from build123d import *

# Parameters (mm, degrees)
SKETCH2_R          = 10
CUT_EXTRUDE1_DEPTH = 216
CUT_EXTRUDE2_DEPTH = 108
CUT_EXTRUDE3_DEPTH = 108
SKETCH7_R          = 15
CUT_EXTRUDE4_DEPTH = 108


with BuildPart() as part:
    # Sketch1 → Revolve1 (revolve)
    with BuildSketch(Plane(origin=(0, 0, 0), x_dir=(1, 0, 0), z_dir=(0, 1, 0)), mode=Mode.PRIVATE) as revolve1_sk:
        Polygon((-1.846866082, -35.985748219), (-1.846866082, 124.014251781), (-46.846866082, 124.014251781), (-46.846866082, 34.014251781), (-31.846866082, 34.014251781), (-31.846866082, -5.985748219), (-21.846866082, -5.985748219), (-21.846866082, -35.985748219), align=None)
    revolve(revolve1_sk.sketch.rotate(Axis((-1.846866082, 0, 35.985748219), (0, 0, -1)), 180), axis=Axis((-1.846866082, 0, 35.985748219), (0, 0, -1)))

    # Sketch2 → Cut-Extrude1 (cut)
    with BuildSketch(Plane.XY.offset(35.985748219)):
        Circle(SKETCH2_R)
    extrude(amount=-CUT_EXTRUDE1_DEPTH, mode=Mode.SUBTRACT)

    # Sketch4 → Cut-Extrude2 (cut, symmetric)
    with BuildSketch(Plane(origin=(0, 0, 0), x_dir=(0, 0, -1), z_dir=(1, 0, 0))):
        with BuildLine():
            Line((124.014251781, 45), (64.014251781, 45))
            Line((64.014251781, 45), (64.014251781, 40))
            ThreePointArc((64.014251781, 40), (66.94318397, 32.928932188), (74.014251781, 30))
            Line((74.014251781, 30), (94.014251781, 30))
            ThreePointArc((94.014251781, 30), (115.227455222, 21.213203431), (124.014251781, -1.4e-08))
            Line((124.014251781, -1.4e-08), (124.014251781, 45))
        make_face()
        with BuildLine():
            Line((124.014251781, -45), (124.014251781, -1.4e-08))
            ThreePointArc((124.014251781, -1.4e-08), (115.227455212, -21.213203441), (94.014251781, -30))
            Line((94.014251781, -30), (74.014251781, -30))
            ThreePointArc((74.014251781, -30), (66.94318397, -32.928932188), (64.014251781, -40))
            Line((64.014251781, -40), (64.014251781, -45))
            Line((64.014251781, -45), (124.014251781, -45))
        make_face()
    extrude(amount=CUT_EXTRUDE2_DEPTH, both=True, mode=Mode.SUBTRACT)

    # Sketch5 → Cut-Extrude3 (cut, symmetric)
    with BuildSketch(Plane(origin=(0, -30, 0), x_dir=(-1, 0, 0), z_dir=(0, -1, 0))):
        with BuildLine():
            Line((-20, 129.367247505), (20, 129.367247505))
            Line((20, 129.367247505), (20, 79.367247505))
            ThreePointArc((20, 79.367247505), (17.071067812, 72.296179693), (10, 69.367247505))
            Line((10, 69.367247505), (-10, 69.367247505))
            ThreePointArc((-10, 69.367247505), (-17.071067812, 72.296179693), (-20, 79.367247505))
            Line((-20, 79.367247505), (-20, 129.367247505))
        make_face()
    extrude(amount=CUT_EXTRUDE3_DEPTH, both=True, mode=Mode.SUBTRACT)

    # Sketch7 → Cut-Extrude4 (cut, symmetric)
    with BuildSketch(Plane(origin=(0, 0, 0), x_dir=(0, 0, -1), z_dir=(1, 0, 0))):
        with Locations((94.014251781, 0)):
            Circle(SKETCH7_R)
    extrude(amount=CUT_EXTRUDE4_DEPTH, both=True, mode=Mode.SUBTRACT)


solid = part.part
Geometry: final body of the model. Coordinates: model frame, mm. A direction names the side the tool comes from. Coordinates: 2 decimals unless noted, no trailing zeros. Loops run counter-clockwise (first coordinate to the right, second up) from the corner with the lowest first, then second, coordinate; pieces in that order, holes last. Notation, with made-up numbers: (45.25, -37) - (89.25, -37) arc R24 cw to (89.25, -13) - close; hole circle Ø5 at (52.25, 31.25). An arc over 180 degrees is marked (long way). One line per question, with ' | ' between items. Start each with the question number.
(1) Reachability of faces 4 (the cylindrical face through (17.23, -6.01, 21.2)), 5 (the flat face through (25, 30, -84)), 6 (the flat face through (20, 0, -111)), 7 (the cylindrical face through (-33.23, 0.66, -79.03)) from +Z, -Z, +X, -X, +Y, -Y: full face, straight path, thin tool, end or side. Return the list, or none.
(2) Cut plane B-B on z = -96.5. Output: boundary loops of the cut face in (x, y), and give its area (3 significant figures).
(3) Cut plane D-D on z = -41. Output: boundary loops of the cut face in (x, y).
(4) Cut plane A-A on x = 1. Output: boundary loops of the cut face in (y, z).
(5) First-contact query: pin 1 (8 mm diameter, centred on y = -23.5, z = -64.5, fed in from +X); pin 2 (10.5 mm diameter, centred on x = 22, z = -83.5, fed in from -Y); pin 3 (1.5 mm diameter, centred on x = -8, y = -42.5, fed in from -Z). Flat tips, straight axial feed; report the tip coordinate or a pass-through.
(6) Ray query, L1, parallel to Z at x = -25, y = 0; L2, parallel to Z at x = -38, y = 0; L3, parallel to Y at x = 29, z = -75. Return the intervals inside material, ascending. Write a range as from..to.
(7) Draft query along Y for faces 1 (the cylindrical face through (39.72, 17.24, -68.38)), 2 (the cylindrical face through (31.736, -13.308, -100.936)), 3 (the flat face through (25, -30, -84)). Return one class per face: +Y half, -Y half, draft (parallel to the pull), parting line (faces both ways), or undercut.
(8) Cut plane C-C on y = -28. Output: boundary loops of the cut face in (x, z), and give its area (3 significant figures).
Here are the results:
1) face 4: +Z | face 5: -Z, +X, -X, +Y | face 6: -Z, +Y, -Y | face 7: +X, -X
2) outline: (-44.35, -14.79) arc R45 ccw to (-35.48, -29.9) - (-20, -29.9) - (-20, -14.79) - close; (-44.35, 14.79) - (-20, 14.79) - (-20, 29.9) - (-35.48, 29.9) arc R45 ccw to start; (20, -29.9) - (31.79, -29.9) arc R45 ccw to (40.65, -14.79) - (20, -14.79) - close; (20, 14.79) - (40.65, 14.79) arc R45 ccw to (31.79, 29.9) - (20, 29.9) - close | area: 1,130 mm²
3) outline: circle Ø90 at (-1.85, 0); hole circle Ø20 at (0, 0)
4) outline: (-44.91, -64.01) - (-40, -64.01) arc R10 cw to (-31.15, -69.37) - (-9.95, -69.37) - (-9.95, 35.99) - (-19.8, 35.99) - (-19.8, 5.99) - (-29.86, 5.99) - (-29.86, -34.01) - (-44.91, -34.01) - close; (9.95, -69.37) - (31.15, -69.37) arc R10 cw to (40, -64.01) - (44.91, -64.01) - (44.91, -34.01) - (29.86, -34.01) - (29.86, 5.99) - (19.8, 5.99) - (19.8, 35.99) - (9.95, 35.99) - close
5) pin 1: x = 38.71 | pin 2: y = -30 | pin 3: z = -64.01
6) L1: -124.01..-109.01, -79.01..5.99 | L2: -124.01..-109.01, -79.01..-34.01 | L3: -30..30
7) face 1: parting line | face 2: undercut | face 3: -Y half
8) outline: (-37.07, -104.78) - (-20, -104.78) - (-20, -79.37) arc R10 cw to (-10, -69.37) - (10, -69.37) arc R10 cw to (20, -79.37) - (20, -104.78) - (33.38, -104.78) - (33.38, -34.01) - (8.92, -34.01) - (8.92, 5.99) - (-12.62, 5.99) - (-12.62, -34.01) - (-37.07, -34.01) - close | area: 4,470 mm²
